```python
from build123d import *

# Parameters (mm, degrees)
SKETCH_1_W           = 75
SKETCH_1_H           = 27
SKETCH_1_R           = 9.5
EXTRUDE_1_DEPTH      = 8
SKETCH_9_R           = 12
CUT_EXTRUDE_7_DEPTH  = 6
SKETCH_11_R          = 1.25
CUT_EXTRUDE_8_DEPTH  = 7
SKETCH_12_R          = 1.25
CUT_EXTRUDE_9_DEPTH  = 7
SKETCH_13_R          = 1.25
CUT_EXTRUDE_10_DEPTH = 6


with BuildPart() as part:
    # Эскиз1 → Бобышка-Вытянуть1 (new body)
    with BuildSketch(Plane(origin=(0, 0, 0), x_dir=(1, 0, 0), z_dir=(0, 1, 0))):
        Rectangle(SKETCH_1_W, SKETCH_1_H)
        with Locations(Location((0, 0, 0), (0, 0, 270))):  # turned: the seam where the file's is
            Circle(SKETCH_1_R, mode=Mode.SUBTRACT)
        with BuildLine():
            Line((-28.5, 9.5), (-22, 9.5))
            ThreePointArc((-22, 9.5), (-18.464466094, 8.035533906), (-17, 4.5))
            Line((-17, 4.5), (-17, -4.5))
            ThreePointArc((-17, -4.5), (-18.464466094, -8.035533906), (-22, -9.5))
            Line((-22, -9.5), (-28.5, -9.5))
            ThreePointArc((-28.5, -9.5), (-32.035533906, -8.035533906), (-33.5, -4.5))
            Line((-33.5, -4.5), (-33.5, 4.5))
            ThreePointArc((-33.5, 4.5), (-32.035533906, 8.035533906), (-28.5, 9.5))
        make_face(mode=Mode.SUBTRACT)
        with BuildLine():
            Line((28.5, 9.5), (22, 9.5))
            ThreePointArc((22, 9.5), (18.464466094, 8.035533906), (17, 4.5))
            Line((17, 4.5), (17, -4.5))
            ThreePointArc((17, -4.5), (18.464466094, -8.035533906), (22, -9.5))
            Line((22, -9.5), (28.5, -9.5))
            ThreePointArc((28.5, -9.5), (32.035533906, -8.035533906), (33.5, -4.5))
            Line((33.5, -4.5), (33.5, 4.5))
            ThreePointArc((33.5, 4.5), (32.035533906, 8.035533906), (28.5, 9.5))
        make_face(mode=Mode.SUBTRACT)
    extrude(amount=EXTRUDE_1_DEPTH)

    # Эскиз9 → Вырез-Вытянуть7 (cut)
    with BuildSketch(Plane.XZ):
        with Locations(Location((0, 0, 0), (0, 0, 270))):  # turned: the seam where the file's is
            Circle(SKETCH_9_R)
    extrude(amount=-CUT_EXTRUDE_7_DEPTH, mode=Mode.SUBTRACT)

    # Эскиз11 → Вырез-Вытянуть8 (cut)
    with BuildSketch(Plane(origin=(0, 0, -13.5), x_dir=(-1, 0, 0), z_dir=(0, 0, -1))):
        with Locations((14.5, 4)):
            Circle(SKETCH_11_R)
        with Locations((33.5, 4)):
            Circle(SKETCH_11_R)
        with Locations(Location((-33.5, 4, 0), (0, 0, 70.49194101))):  # turned: the seam where the file's is
            Circle(SKETCH_11_R)
        with Locations(Location((-14.5, 4, 0), (0, 0, 180))):  # turned: the seam where the file's is
            Circle(SKETCH_11_R)
    extrude(amount=-CUT_EXTRUDE_8_DEPTH, mode=Mode.SUBTRACT)

    # Эскиз12 → Вырез-Вытянуть9 (cut)
    with BuildSketch(Plane.XY.offset(13.5)):
        with Locations(Location((-14.5, 4, 0), (0, 0, 180))):  # turned: the seam where the file's is
            Circle(SKETCH_12_R)
        with Locations(Location((-33.5, 4, 0), (0, 0, 180))):  # turned: the seam where the file's is
            Circle(SKETCH_12_R)
        with Locations((14.5, 4)):
            Circle(SKETCH_12_R)
        with Locations(Location((33.5, 4, 0), (0, 0, 109.50805899))):  # turned: the seam where the file's is
            Circle(SKETCH_12_R)
    extrude(amount=-CUT_EXTRUDE_9_DEPTH, mode=Mode.SUBTRACT)

    # Эскиз13 → Вырез-Вытянуть10 (cut)
    with BuildSketch(Plane.XZ):
        with Locations(Location((-11.29380733, 9.083435331, 0), (0, 0, 270))):  # turned: the seam where the file's is
            Circle(SKETCH_13_R)
        with Locations(Location((11.29380733, 9.083435331, 0), (0, 0, 90))):  # turned: the seam where the file's is
            Circle(SKETCH_13_R)
        with Locations(Location((11.29380733, -9.083435331, 0), (0, 0, 270))):  # turned: the seam where the file's is
            Circle(SKETCH_13_R)
        with Locations(Location((-11.29380733, -9.083435331, 0), (0, 0, 90))):  # turned: the seam where the file's is
            Circle(SKETCH_13_R)
    extrude(amount=-CUT_EXTRUDE_10_DEPTH, mode=Mode.SUBTRACT)


solid = part.part
```
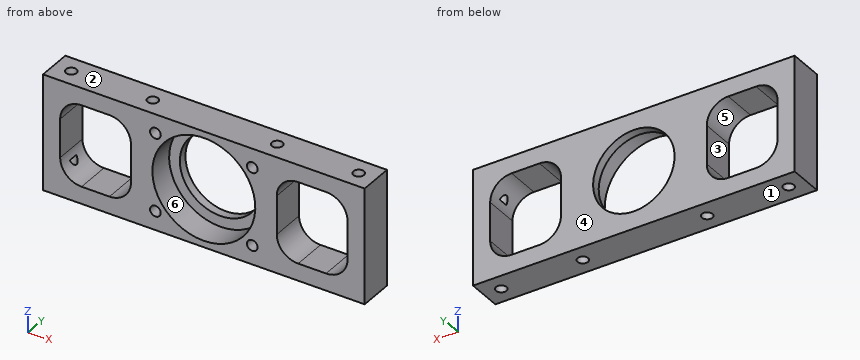
Work out the finished part from the listing and answer in its coordinate system (mm). Face numbers are marked on the shaded views. A direction names the side the tool comes from. Round coordinates to 2 decimals unless told otherwise and drop trailing zeros. Order: outer loops, then holes, each group sorted by start corner. A loop starts at its lowest first (then second) coordinate and runs counter-clockwise, first axis right, second up.
Q1. Given pin 1 Ø0.8 at (x, y) = (14, 3.5) entering from -Z; pin 2 Ø3 at (x, y) = (-15, 4) entering from -Z; pin 3 Ø0.8 at (x, y) = (-14.5, 4.5) entering from +Z; pin 4 Ø12 at (x, z) = (5, -1) entering from -Y, each flat-ended and moving along its own axis, determine where each tip first touches the part or whether it passes through.
Solution:
pin 1: stops at z = -6.5
pin 2: stops at z = -13.5
pin 3: stops at z = 6.5
pin 4: stops at y = 6
Q2. The mould has two halves that part along Z. Classify the marked faces 1, 2 and 3: pulls with the +Z half, pulls with the -Z half, needs draft (parallel to the pull), parting line crosses it, or undercut.
Solution:
face 1: pulls with the -Z half
face 2: pulls with the +Z half
face 3: undercut
Q3. A tool of negligible diameter and unlimited length cuts with its end or side. For the marked faces 4, 5 and 6, from which of +Z, -Z, +X, -X, +Y, -Y can it reach the whole face along a straight path? Write none if from no direction.
Solution:
face 4: +Z, -Z, +X, -X, +Y
face 5: +Y, -Y
face 6: -Y
Q4. A cutting plane is placed at C-C, the plane x = 14.5. Determine the outline of the cut face in (y, z), then the cut area to 3 significant figures.
Solution:
outline: (0, -13.5) - (2.75, -13.5) - (2.75, -6.5) - (5.25, -6.5) - (5.25, -13.5) - (8, -13.5) - (8, 13.5) - (5.25, 13.5) - (5.25, 6.5) - (2.75, 6.5) - (2.75, 13.5) - (0, 13.5) - close
area: 181 mm2
Q5. Find the intervals of material crossed by line 1 along X through (y, z) = (6.4, 0); line 2 along Z through (x, y) = (-27, 2.5); line 3 along X through (y, z) = (4, -2.5), in increasing order.
Solution:
line 1: x = -37.5 to -33.5, -17 to -9.5, 9.5 to 17, 33.5 to 37.5
line 2: z = -13.5 to -9.5, 9.5 to 13.5
line 3: x = -37.5 to -33.5, -17 to -11.74, 11.74 to 17, 33.5 to 37.5
Q6. A cutting plane is placed at B-B, the plane z = 0. Determine the outline of the cut face in (x, y), then the cut area to 3 significant figures.
Solution:
outline: (-37.5, 0) - (-33.5, 0) - (-33.5, 8) - (-37.5, 8) - close; (-17, 0) - (-12, 0) - (-12, 6) - (-9.5, 6) - (-9.5, 8) - (-17, 8) - close; (9.5, 6) - (12, 6) - (12, 0) - (17, 0) - (17, 8) - (9.5, 8) - close; (33.5, 0) - (37.5, 0) - (37.5, 8) - (33.5, 8) - close
area: 154 mm2
Q7. A cutting plane is placed at A-A, the plane x = 26. Determine the outline of the cut face in (y, z).
Solution:
outline: (0, -13.5) - (8, -13.5) - (8, -9.5) - (0, -9.5) - close; (0, 9.5) - (8, 9.5) - (8, 13.5) - (0, 13.5) - close
Q8. A cutting plane is placed at D-D, the plane y = 2. Determine the outline of the cut face in (x, z).
Solution:
outline: (-37.5, -13.5) - (37.5, -13.5) - (37.5, 13.5) - (-37.5, 13.5) - close; hole (-33.5, -4.5) arc R5 ccw to (-28.5, -9.5) - (-22, -9.5) arc R5 ccw to (-17, -4.5) - (-17, 4.5) arc R5 ccw to (-22, 9.5) - (-28.5, 9.5) arc R5 ccw to (-33.5, 4.5) - close; hole circle Ø2.5 at (-11.29, -9.08); hole circle Ø2.5 at (-11.29, 9.08); hole circle Ø24 at (0, 0); hole circle Ø2.5 at (11.29, -9.08); hole circle Ø2.5 at (11.29, 9.08); hole (17, -4.5) arc R5 ccw to (22, -9.5) - (28.5, -9.5) arc R5 ccw to (33.5, -4.5) - (33.5, 4.5) arc R5 ccw to (28.5, 9.5) - (22, 9.5) arc R5 ccw to (17, 4.5) - close
